Read the model definition and answer for the solid it produces. Units are mm, in the model's axes. Coordinates: 2 decimals unless noted, no trailing zeros. Order: outer loops, then holes, each group sorted by start corner. A loop starts at its lowest first (then second) coordinate and runs counter-clockwise, first axis right, second up.
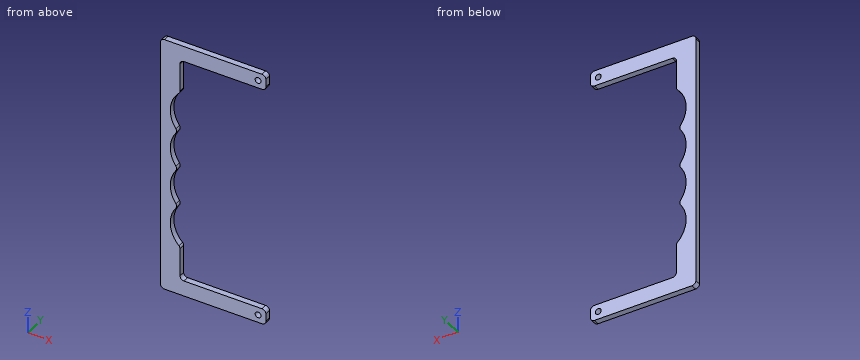
Autodesk Inventor part; units mm, degrees
ref_plane "YZ Plane" through (0, 0, 0) normal (1, 0, 0) x (0, 1, 0)
ref_plane "XZ Plane" through (0, 0, 0) normal (0, 1, 0) x (-1, 0, 0)
ref_plane "XY Plane" through (0, 0, 0) normal (0, 0, 1) x (1, 0, 0)
sketch "Sketch1" plane through (0, 0, 0) normal (0, 1, 0) x (-1, 0, 0)
  line L0 (0, 0) -> (50, 0) construction
  line L1 (0, 0) -> (0, -62.5) construction
  line L2 (0, -62.5) -> (-4, -62.5) construction
  line L3 (40, -58.5) -> (-4, -58.5)
  line L4 (-4, -58.5) -> (-4, -66.5)
  line L5 (-4, -66.5) -> (50, -66.5)
  line L6 (50, -66.5) -> (50, 66.5)
  line L7 (50, 66.5) -> (-4, 66.5)
  line L8 (-4, 66.5) -> (-4, 58.5)
  line L9 (-4, 58.5) -> (40, 58.5)
  line L10 (40, 58.5) -> (40, -58.5)
  point P0 (0, 62.5)
  dimension "d0" = 62.5
  dimension "d1" = 50
  dimension "d2" = 4
  dimension "d3" = 8
  dimension "d4" = 10
extrude "Plate1" add sketch "Sketch1" along normal blind 3
hole "Hole1" at (0, 0, -62.5) at (0, 0, 62.5) direction (0, 1, 0) diameter 3 end through all
sketch "Sketch2" plane through (0, 3, 0) normal (0, 1, 0) x (1, 0, 0)
  circle A0 centre (0, 62.5) radius 1.5
  circle A1 centre (0, -62.5) radius 1.5
  line L0 (-40, 58.5) -> (-40, -58.5)
  line L1 (4, 58.5) -> (-40, 58.5)
  line L2 (4, 66.5) -> (4, 58.5)
  line L3 (-50, 66.5) -> (4, 66.5)
  line L4 (-50, -66.5) -> (-50, 66.5)
  line L5 (4, -66.5) -> (-50, -66.5)
  line L6 (4, -58.5) -> (4, -66.5)
  line L7 (-40, -58.5) -> (4, -58.5)
  circle A2 centre (-30, -30) radius 15
  circle A3 centre (-30, -10) radius 15
  circle A4 centre (-30, 10) radius 15
  circle A5 centre (-30, 30) radius 15
  line L8 (-30, 30) -> (-30, -30) construction
  line L9 (-30, 30) -> (-30, 58.5) construction
  line L10 (-30, -30) -> (-30, -58.5) construction
  point P0 (0, 0)
  dimension "d13" = 20
  dimension "d14" = 20
  dimension "d15" = 30
  dimension "d16" = 20
  dimension "d17" = 10
extrude "Extrusion1" cut sketch "Sketch2" against normal through all contours A5 A4 L0 | L0 A4 A5 | A4 A5 L0 | L0 A5 A4 | A5 L0 A3 A4 | A5 A4 A3 L0 | A4 L0 A2 A3 | A3 L0 A4 | A3 A4 L0 | A3 L0 A2 | A2 L0 A3 | A4 A3 A2 L0 | A2 A3 L0 | L0 A3 A2
fillet "Fillet1" radius 2 8 edges at (-50, 1.5, 66.5) (-40, 1.5, 58.5) (4, 1.5, 66.5) (4, 1.5, 58.5) (4, 1.5, -58.5) (4, 1.5, -66.5) (-40, 1.5, -58.5) (-50, 1.5, -66.5)
fillet "Fillet2" radius 2 5 edges at (-40, 1.5, 41.1803) (-41.1803, 1.5, 20) (-41.1803, 1.5, 0) (-41.1803, 1.5, -20) (-40, 1.5, -41.1803)
equation "\"d0\" = 0.5 * holes_spacing"
equation "\"d1\" = handle_height"
equation "\"d2\" = hole_2_border"
equation "\"d3\" = 2 * hole_2_border"
equation "\"d4\" = handle_width"
equation "\"d11\" = Thickness"
equation "\"d13\" = finger_trace_width"
equation "\"d14\" = finger_trace_width"
equation "\"d15\" = finger_trace_diameter"
equation "\"d16\" = finger_trace_width"
equation "\"d5\" = Thickness"
equation "\"hole_2_border\" = 4"
equation "\"BendRadius\" = Thickness"
equation "\"BendReliefWidth\" = Thickness"
equation "\"BendReliefDepth\" = 0.5 * Thickness"
equation "\"CornerReliefSize\" = 4 * Thickness"
equation "\"MinimumRemnant\" = 2 * Thickness"
equation "\"TransitionRadius\" = BendRadius"
equation "\"JacobiRadiusSize\" = BendRadius"
equation "\"GapSize\" = Thickness"
equation "\"handle_height\" = 50"
equation "\"handle_width\" = 10"
equation "\"finger_trace_diameter\" = 30"
equation "\"finger_trace_width\" = 20"
properties part number "handle_v3"
1) A cutting plane is placed at B-B, the plane z = -62.5. Determine the outline of the cut face in (x, y), and give its area (3 significant figures).
A:
outline: (-50, 0) - (-1.5, 0) - (-1.5, 3) - (-50, 3) - close; (1.5, 0) - (4, 0) - (4, 3) - (1.5, 3) - close
area: 153 mm2
2) A cutting plane is placed at A-A, the plane x = -9.5. Determine the outline of the cut face in (y, z).
A:
outline: (0, -66.5) - (3, -66.5) - (3, -58.5) - (0, -58.5) - close; (0, 58.5) - (3, 58.5) - (3, 66.5) - (0, 66.5) - close
3) Straight lines are drawn through the part: line 1 (Z direction, x = 0, y = 1.65); line 2 (Z direction, x = -29, y = 1.2); line 3 (X direction, y = 1.4, z = 62.5). For each, find the intervals that lie inside material, in ascending order.
A:
line 1: z = -66.5 to -64, -61 to -58.5, 58.5 to 61, 64 to 66.5
line 2: z = -66.5 to -58.5, 58.5 to 66.5
line 3: x = -50 to -1.5, 1.5 to 4
4) A cutting plane is placed at C-C, the plane x = 0. Determine the outline of the cut face in (y, z), and give its area (3 significant figures).
A:
outline: (0, -66.5) - (3, -66.5) - (3, -64) - (0, -64) - close; (0, -61) - (3, -61) - (3, -58.5) - (0, -58.5) - close; (0, 58.5) - (3, 58.5) - (3, 61) - (0, 61) - close; (0, 64) - (3, 64) - (3, 66.5) - (0, 66.5) - close
area: 30.0 mm2
5) A cutting plane is placed at D-D, the plane z = -30. Determine the outline of the cut face in (x, y), and give its area (3 significant figures).
A:
outline: (-50, 0) - (-45, 0) - (-45, 3) - (-50, 3) - close
area: 15.0 mm2
6) Flat-ended cylindrical pins translate along their axes: pin 1 Ø1.8 at (x, z) = (0, 62.5) entering from +Y; pin 2 Ø1.5 at (y, z) = (2, -46) entering from +X. Find the tip coordinate at first contact, or state that the pin passes through.
A:
pin 1: passes through
pin 2: stops at x = -40
